Here's the drawing with two shaded views (mm, measured from the low corner). I have some questions. A direction names the side the tool comes from. Coordinates: 2 decimals unless noted, no trailing zeros. Write each loop counter-clockwise with the first axis right and the second up, starting at its lowest first coordinate (ties: lowest second). Pieces come first, ordered by that corner, then holes. Notation, with made-up numbers: (-0.75, 58.25) -> (22.25, 58.25) arc R11 ccw to (22.25, 79.25) -> close; hole circle Ø2 at (77, 20). An arc over 180 degrees is marked (long way). Use one line per item in the form item = value.
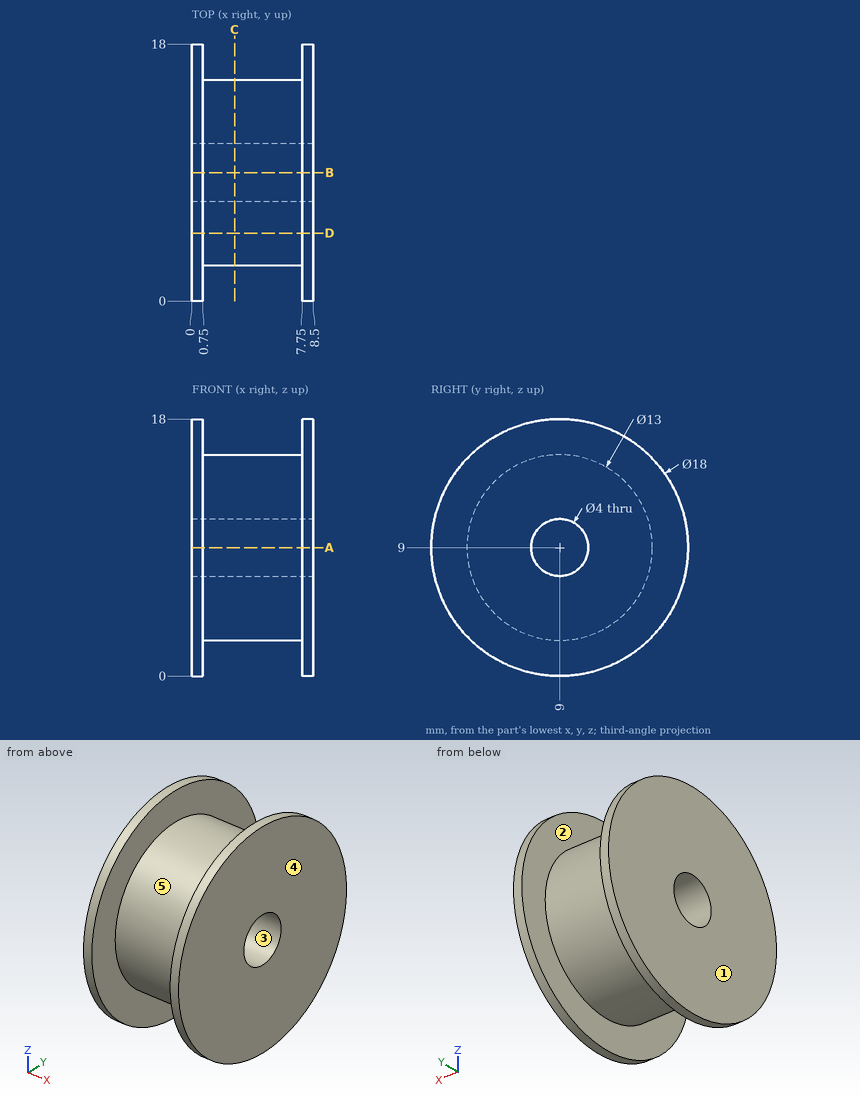
Q1. If I drill on line 1 (X direction, y = 2.75, z = 15); line 2 (Z direction, x = 5.75, y = 9); line 3 (Z direction, x = 1.5, y = 10.25), over which ranges is the centre line in solid material (lowest first)? Write a range as from..to.
Return value:
line_1 = 0..0.75, 7.75..8.5
line_2 = 2.5..7, 11..15.5
line_3 = 2.62..7.44, 10.56..15.38
Q2. Will these pins go through, and if not, where does the flat tip stop? pin 1 (5 mm diameter, centred on x = 2, z = 2.5, fed in from -Y); pin 2 (1.5 mm diameter, centred on x = 4.5, y = 3.5, fed in from -Z); pin 3 (3 mm diameter, centred on y = 9, z = 9, fed in from +X); pin 4 (4 mm diameter, centred on x = 1, z = 15.5, fed in from -Y).
Return value:
pin_1 = 1.11
pin_2 = 4.56
pin_3 = through
pin_4 = 1.21
Q3. For the marked faces 1 and 2, which set-ups out of +Z, -Z, +X, -X, +Y, -Y let a thin tool reach every point of the face, with its end or its side?
Return value:
face_1 = +Z, -Z, -X, +Y, -Y
face_2 = none
Q4. Thinking about a two-plate mould opening in X: for the marked faces 3, 4 and 5, which applies, released by +X, released by -X, zero draft, split by the parting line, or undercut?
Return value:
face_3 = zero draft
face_4 = released by +X
face_5 = undercut
Q5. Suppose I cut it at D-D (y = 4.75). Write out the boundary of the cut face in (x, z).
Return value:
outline = (0, 1.07) -> (0.75, 1.07) -> (0.75, 4.08) -> (7.75, 4.08) -> (7.75, 1.07) -> (8.5, 1.07) -> (8.5, 16.93) -> (7.75, 16.93) -> (7.75, 13.92) -> (0.75, 13.92) -> (0.75, 16.93) -> (0, 16.93) -> close
Q6. Suppose I cut it at A-A (z = 9). Write out the boundary of the cut face in (x, y).
Return value:
outline = (0, 0) -> (0.75, 0) -> (0.75, 2.5) -> (7.75, 2.5) -> (7.75, 0) -> (8.5, 0) -> (8.5, 7) -> (0, 7) -> close; (0, 11) -> (8.5, 11) -> (8.5, 18) -> (7.75, 18) -> (7.75, 15.5) -> (0.75, 15.5) -> (0.75, 18) -> (0, 18) -> close
Q7. Suppose I cut it at C-C (x = 3). Write out the boundary of the cut face in (y, z).
Return value:
outline = circle Ø13 at (9, 9); hole circle Ø4 at (9, 9)
